from build123d import *

# Parameters (mm, degrees)
ESQUISSE1_R             = 0.750000000000002
ESQUISSE1_R_2           = 1.05
BOSS_EXTRU_1_DEPTH      = 5.588
BOSS_EXTRU_2_DEPTH      = 8.889999999999999
ENL_V_MAT_EXTRU_1_DEPTH = 2.5
ESQUISSE4_R             = 1.05
ENL_V_MAT_EXTRU_2_DEPTH = 51.616470975365324
CONG_1_R                = 5.588
CONG_2_R                = 2.54


with BuildPart() as part:
    # Esquisse1 → Boss.-Extru.1 (new body)
    with BuildSketch(Plane(origin=(0, 0, 0), x_dir=(0, 0, -1), z_dir=(1, 0, 0))):
        with BuildLine():
            ThreePointArc((-28.574999999999996, 0), (-22.86, 17.144999999999996), (-8.00099999999999, 27.432000000000002))
            ThreePointArc((-8.00099999999999, 27.432000000000002), (-5.841999999999989, 31.369000000000003), (-9.778999999999986, 33.528))
            ThreePointArc((-9.778999999999986, 33.528), (-27.939999999999998, 20.955), (-34.925, 0))
            ThreePointArc((-34.925, 0), (-31.75, -3.174999999999997), (-28.574999999999996, 0))
        make_face()
        with Locations((-31.75, 0)):
            Circle(ESQUISSE1_R, mode=Mode.SUBTRACT)
        with Locations((-8.889999999999992, 30.480000000000004)):
            Circle(ESQUISSE1_R_2, mode=Mode.SUBTRACT)
    extrude(amount=BOSS_EXTRU_1_DEPTH)

    # Esquisse2 → Boss.-Extru.2 (add)
    with BuildSketch(Plane(origin=(5.588, 0, 0), x_dir=(0, 0, -1), z_dir=(1, 0, 0))):
        with BuildLine():
            Line((-15.468698222001095, 24.026027560057866), (-18.836262664685126, 29.410046477810756))
            ThreePointArc((-18.836262664685126, 29.410046477810756), (-14.455023336022604, 31.793205647670106), (-9.778999999999986, 33.528000000000006))
            ThreePointArc((-9.778999999999986, 33.528000000000006), (-5.8419999999999845, 31.369000000000003), (-8.000999999999987, 27.432))
            ThreePointArc((-8.000999999999987, 27.432), (-11.85777574941277, 25.9985341755384), (-15.468698222001095, 24.026027560057866))
        make_face()
    extrude(amount=BOSS_EXTRU_2_DEPTH)

    # Esquisse3 → Enlèv. mat.-Extru.1 (cut, symmetric)
    with BuildSketch(Plane(origin=(9.487780000000024, 4.74e-15, -3.69e-15), x_dir=(-1.3e-16, 0, -1), z_dir=(1, 2.5e-16, -1.3e-16))):
        with BuildLine():
            Line((-11.857775749412772, 25.9985341755384), (-14.455023336022602, 31.793205647670096))
            ThreePointArc((-14.455023336022602, 31.793205647670096), (-12.148018341439107, 32.74417925946624), (-9.778999999999993, 33.528))
            ThreePointArc((-9.778999999999993, 33.528), (-5.84199999999999, 31.368999999999996), (-8.000999999999994, 27.43199999999999))
            ThreePointArc((-8.000999999999994, 27.43199999999999), (-9.9552222292544, 26.78477506655896), (-11.857775749412772, 25.9985341755384))
        make_face()
    extrude(amount=ENL_V_MAT_EXTRU_1_DEPTH, both=True, mode=Mode.SUBTRACT)

    # Esquisse4 → Enlèv. mat.-Extru.2 (cut, through all)
    with BuildSketch(Plane.ZY):
        with Locations(Location((8.889999999999992, 30.480000000000004, 0), (0, 0, 90))):
            Circle(ESQUISSE4_R)
    extrude(amount=-ENL_V_MAT_EXTRU_2_DEPTH, mode=Mode.SUBTRACT)

    # Congé1
    cong_1_edges = [part.edges().sort_by_distance(p)[0] for p in [
        (5.588, 26.71803701893431, 17.152480443343112),
    ]]
    fillet(cong_1_edges, radius=CONG_1_R)

    # Congé2
    cong_2_edges = [part.edges().sort_by_distance(p)[0] for p in [
        (14.477999999999998, 26.71803701893431, 17.152480443343112),
    ]]
    fillet(cong_2_edges, radius=CONG_2_R)


solid = part.part
Check sheet for the modelled part. Datum: model origin and axes. Units: mm. A direction names the side the tool comes from. Round coordinates to 2 decimals unless told otherwise and drop trailing zeros. Loops run counter-clockwise (first coordinate to the right, second up) from the corner with the lowest first, then second, coordinate; pieces in that order, holes last. Notation, with made-up numbers: M -14,16.5 L 28,16.5 A20 cw 28,34.5 Z; hole C 65.25,44.25 d6. An arc over 180 degrees is marked long. One line per question, with ' | ' between items. Start each with the question number.
Item 1: Section check B-B (x = 2). Record the boundary of the cut face in (y, z) (3 decimals).
Item 2: Set-up check for faces 4 (the face through (11.55, 26.68, 17.13)), 5 (the face through (2.755, -3.174, 31.82)), 6 (the face through (11.988, 30, 10)): record each of +Z, -Z, +X, -X, +Y, -Y from which the full face is reachable in a straight line by a thin tool's end or side.
Item 3: Release check for a two-part mould opening along Z. For faces 1 (the face through (3.92, 20.7, 28.13)), 2 (the face through (14.478, 30, 11)), 3 (the face through (13.22, 31.45, 9.29)) record: released by +Z, released by -Z, zero draft, split by the parting line, or undercut.
Item 4: Gauge pin test, flat ends, axial feed: pin 1 Ø8 at (y, z) = (12, 31.5) entering from +X; pin 2 Ø1.5 at (x, z) = (3.5, 22.5) entering from -Y. Record the tip position at first contact, or that the pin passes through.
Item 5: Section check A-A (z = 31.75). Record the boundary of the cut face in (x, y) (3 decimals), and give its area (3 significant figures).
Item 6: Section check D-D (y = 7.5). Record the boundary of the cut face in (x, z).
Item 7: Scan lines: probe 1 along Z at (x, y) = (6.7, 30.48) (3 decimals); probe 2 along Y at (x, z) = (2.75, 8.89) (3 decimals); probe 3 along X at (y, z) = (18, 28.5). Record each from-to range of solid material in increasing order.
Worked out:
1) outline: M 0,28.575 A28.575 cw 27.432,8.001 A3.175 ccw 33.528,9.779 A34.925 ccw 0,34.925 A3.175 ccw Z; hole C 0,31.75 d1.5; hole C 30.48,8.89 d2.1
2) face 4: +Z, +X, -Y | face 5: +X, -X, -Y | face 6: -Z, +Y
3) face 1: released by +Z | face 2: zero draft | face 3: undercut
4) pin 1: x = 5.59 | pin 2: y = 16.61
5) outline: M 0,-3.175 L 5.588,-3.175 L 5.588,-0.75 L 0,-0.75 Z; M 0,0.75 L 5.588,0.75 L 5.588,14.55 L 0,14.55 Z | area: 90.7 mm^2
6) outline: M 0,27.57 L 5.59,27.57 L 5.59,34.11 L 0,34.11 Z
7) probe 1: 5.715 to 7.84, 9.94 to 17.051 | probe 2: 27.157 to 29.43, 31.53 to 33.655 | probe 3: 0 to 5.59
